Can you work these out from the drawing? Everything is in mm from the part's minimum corner. Coordinates: 2 decimals unless noted, no trailing zeros. Write each loop counter-clockwise with the first axis right and the second up, starting at its lowest first coordinate (ties: lowest second). Pieces come first, ordered by that corner, then holes.
(1) Imagine slicing it at D-D, the plane y = 12. List the corners of the cut face in (x, z) for me.
(2) Please list where these lines run through material, in increasing order: probe 1 along Y at (x, z) = (27, 120) (3 decimals); probe 2 along Z at (x, y) = (40.5, 19.05) (3 decimals); probe 3 along Z at (x, y) = (23, 15.75).
(3) Imagine slicing it at B-B, the plane y = 19.05. List the corners of the cut face in (x, z) for me (3 decimals).
(4) Imagine slicing it at C-C, the plane x = 16. List the corners of the cut face in (y, z) for me (3 decimals), plus the area to 3 significant figures.
(5) For pin 1 Ø2 at (x, y) = (14.5, 3.5) entering from -Z; pin 2 Ø3 at (x, y) = (11, 22.5) entering from -Z, each with a flat end and sliding along its axis, tell me the tip position at first contact or that it passes through.
(6) Imagine slicing it at A-A, the plane z = 120.65. List the corners of the cut face in (x, y) for me (3 decimals).
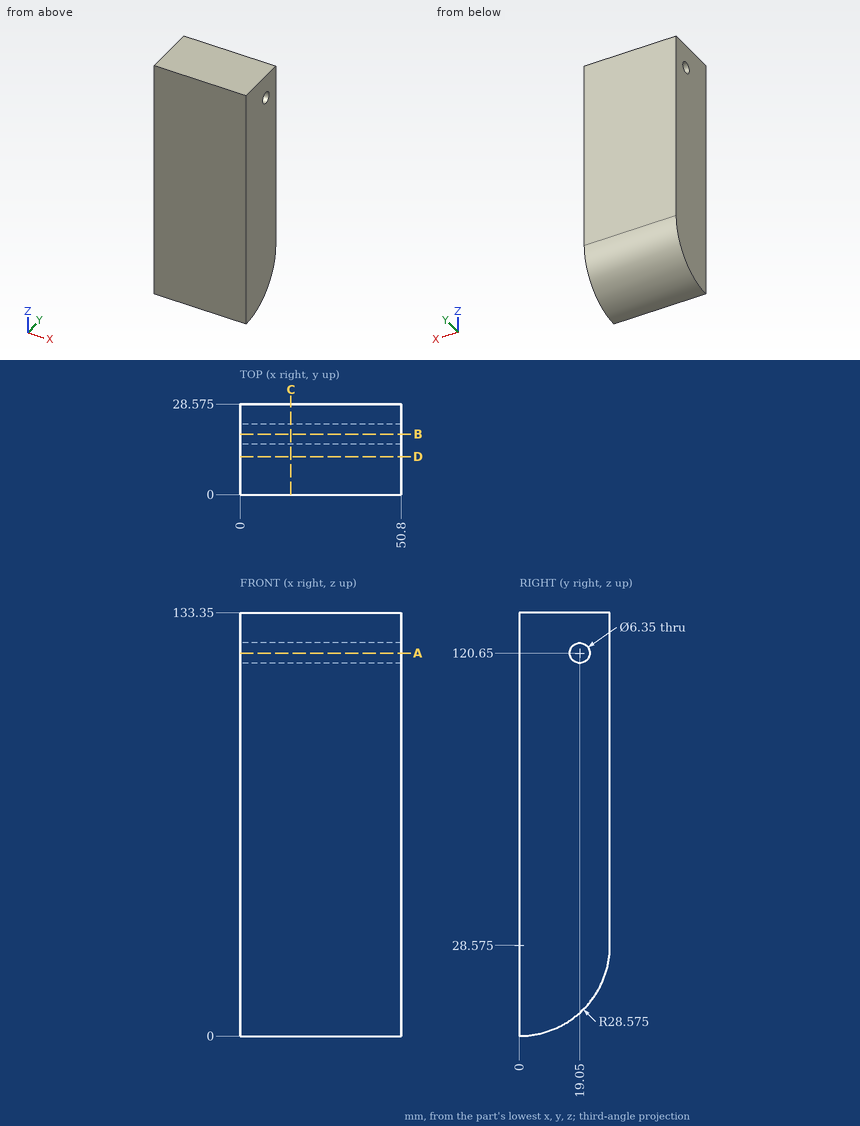
Recorded:
1. outline: (0, 2.64) - (50.8, 2.64) - (50.8, 133.35) - (0, 133.35) - close
2. probe 1: y = 0 to 15.942, 22.158 to 28.575
2. probe 2: z = 7.276 to 117.475, 123.825 to 133.35
2. probe 3: z = 4.73 to 133.35
3. outline: (0, 7.276) - (50.8, 7.276) - (50.8, 117.475) - (0, 117.475) - close; (0, 123.825) - (50.8, 123.825) - (50.8, 133.35) - (0, 133.35) - close
4. outline: (0, 0) arc R28.575 ccw to (28.575, 28.575) - (28.575, 133.35) - (0, 133.35) - close; hole circle Ø6.35 at (19.05, 120.65)
4. area: 3,600 mm2
5. pin 1: stops at z = 0.11
5. pin 2: stops at z = 9.2
6. outline: (0, 0) - (50.8, 0) - (50.8, 15.875) - (0, 15.875) - close; (0, 22.225) - (50.8, 22.225) - (50.8, 28.575) - (0, 28.575) - close
